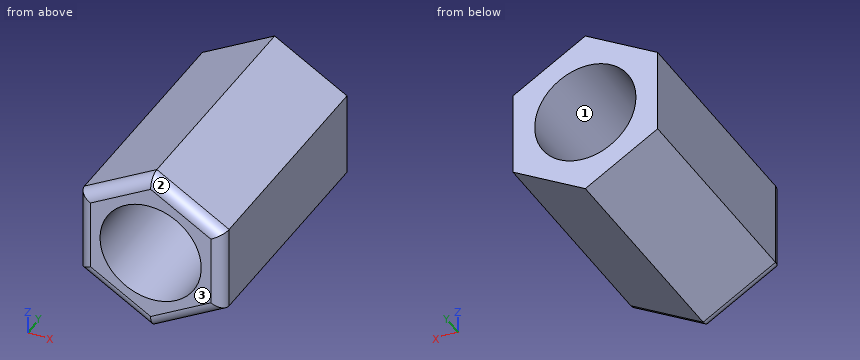
Autodesk Inventor part; units mm, degrees
ref_plane "YZ Plane" through (0, 0, 0) normal (1, 0, 0) x (0, 1, 0)
ref_plane "XZ Plane" through (0, 0, 0) normal (0, 1, 0) x (-1, 0, 0)
ref_plane "XY Plane" through (0, 0, 0) normal (0, 0, 1) x (1, 0, 0)
sketch "Sketch1" plane through (0, 0, 0) normal (0, 1, 0) x (-1, 0, 0)
  circle A0 centre (0, 0) radius 2.1
  line L0 (0, -3.4641) -> (-3, -1.7321)
  line L1 (-3, -1.7321) -> (-3, 1.7321)
  line L2 (-3, 1.7321) -> (0, 3.4641)
  line L3 (0, 3.4641) -> (3, 1.7321)
  line L4 (3, 1.7321) -> (3, -1.7321)
  line L5 (3, -1.7321) -> (0, -3.4641)
  dimension "d0" = 4.2
  dimension "d1" = 3
extrude "Extrusion1" add sketch "Sketch1" along normal blind 10
fillet "Fillet1" radius 0.5 6 edges at (1.5, 0, 2.5981) (3, 0, 0) (-1.5, 0, 2.5981) (-3, 0, 0) (-1.5, 0, -2.5981) (1.5, 0, -2.5981)
thread "Thread1"
properties part number "liftmotorbasenut" material "Iron, Ductile"
Read the model definition and answer for the solid it produces. Units are mm, in the model's axes. Face numbers are marked on the shaded views. Give positions to 0.01 mm unless a question says otherwise; leave off trailing zeros. Loops run counter-clockwise (first coordinate to the right, second up) from the corner with the lowest first, then second, coordinate; pieces in that order, holes last. Notation, with made-up numbers: (74.5, 56) -> (84.5, 56) arc R17 ccw to (84.5, 81) -> close; hole circle Ø4 at (16.5, -16.75). An arc over 180 degrees is marked (long way). Answer as CSV lines item,"result".
Item 1: Determine the mould class of the marked faces 1, 2 and 3 for opening direction Z: +Z half, -Z half, draft (parallel to the pull), parting line (faces both ways), or undercut.
Returned:
face 1,"undercut"
face 2,"+Z half"
face 3,"draft"
Item 2: Find section A-A on z = 0. Give the vertices of the cut face in (x, y), plus the area to 3 significant figures.
Returned:
outline,"(-3, 0.5) arc R0.5 ccw to (-2.5, 0) -> (-2.1, 0) -> (-2.1, 10) -> (-3, 10) -> close; (2.1, 0) -> (2.5, 0) arc R0.5 ccw to (3, 0.5) -> (3, 10) -> (2.1, 10) -> close"
area,"17.9 mm²"
Item 3: Each of these flat-tipped pins is pushed along its axis until it touches: pin 1 (3.5 mm diameter, centred on x = 0, z = 0, fed in from -Y); pin 2 (1.5 mm diameter, centred on x = -1, z = -2.5, fed in from -Y); pin 3 (2 mm diameter, centred on x = -2, y = 1.5, fed in from -Z); pin 4 (2 mm diameter, centred on x = 0.5, y = 5, fed in from -Z). Where does it stop, or does it pass through?
Returned:
pin 1,"passes through"
pin 2,"stops at y = 0"
pin 3,"stops at z = -2.89"
pin 4,"stops at z = -3.46"
Item 4: Consider line 1 (Z direction, x = 1.4, y = 4.25); line 2 (Z direction, x = -1.45, y = 8.75); line 3 (X direction, y = 8.75, z = -0.5). Determine where each line is inside the solid, lowest interval first. Write a range as [from, to].
Returned:
line 1,"z = [-2.66, -1.57], [1.57, 2.66]"
line 2,"z = [-2.63, -1.52], [1.52, 2.63]"
line 3,"x = [-3, -2.04], [2.04, 3]"
Item 5: Find section B-B on y = 6. Give the vertices of the cut face in (x, z).
Returned:
outline,"(-3, -1.73) -> (0, -3.46) -> (3, -1.73) -> (3, 1.73) -> (0, 3.46) -> (-3, 1.73) -> close; hole circle Ø4.2 at (0, 0)"
Item 6: Find section C-C on z = -1. Give the vertices of the cut face in (x, y), plus the area to 3 significant figures.
Returned:
outline,"(-3, 0.5) arc R0.5 ccw to (-2.5, 0) -> (-1.85, 0) -> (-1.85, 10) -> (-3, 10) -> close; (1.85, 0) -> (2.5, 0) arc R0.5 ccw to (3, 0.5) -> (3, 10) -> (1.85, 10) -> close"
area,"23.0 mm²"
